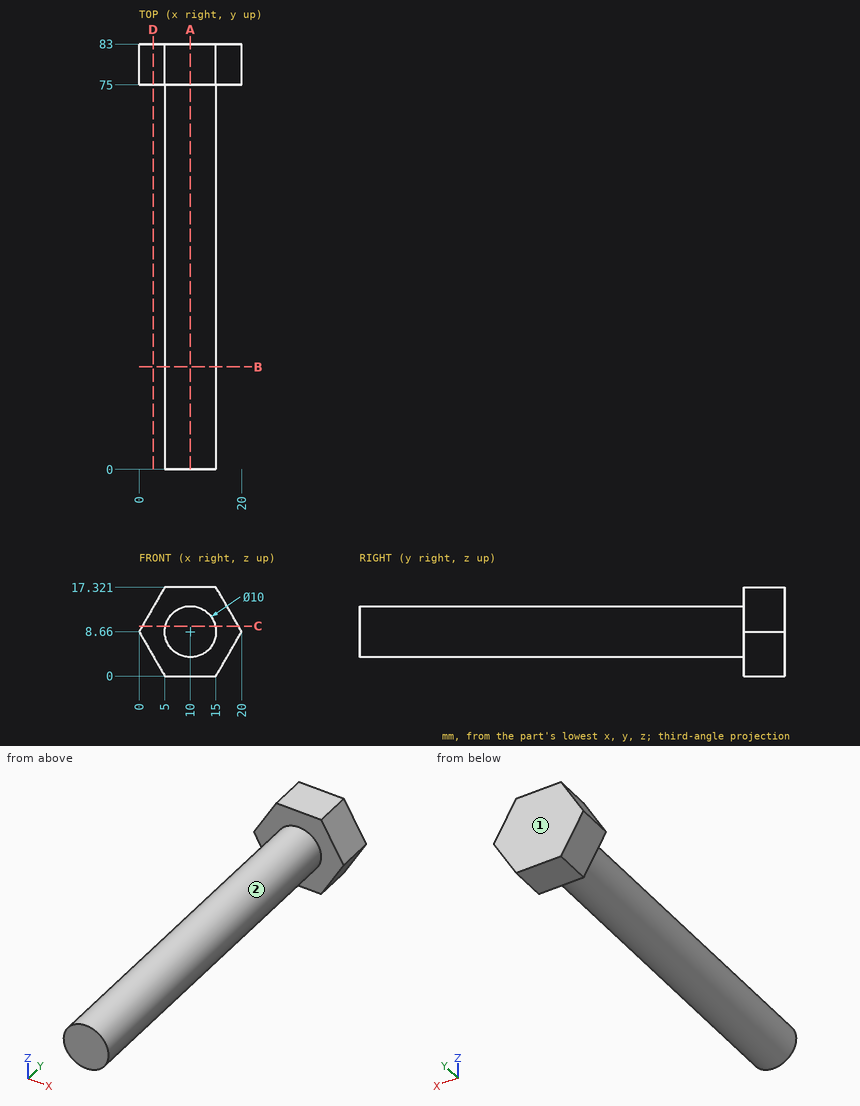
The drawing under review shows one solid part. Ordinate dimensions are in mm from its lowest x, y, z. A direction names the side the tool comes from. Round coordinates to 2 decimals unless told otherwise and drop trailing zeros. Loops run counter-clockwise (first coordinate to the right, second up) from the corner with the lowest first, then second, coordinate; pieces in that order, holes last.
Item 1: Take a section at C-C (z = 9.75). Write out the cut boundary in (x, y), then the cut area to 3 significant figures.
Determined:
outline: (0.63, 75) - (5.12, 75) - (5.12, 0) - (14.88, 0) - (14.88, 75) - (19.37, 75) - (19.37, 83) - (0.63, 83) - close
area: 882 mm2
Item 2: Take a section at A-A (x = 10). Write out the cut boundary in (y, z).
Determined:
outline: (0, 3.66) - (75, 3.66) - (75, 0) - (83, 0) - (83, 17.32) - (75, 17.32) - (75, 13.66) - (0, 13.66) - close
Item 3: Take a section at B-B (y = 20). Write out the cut boundary in (x, z).
Determined:
outline: circle Ø10 at (10, 8.66)
Item 4: Clearance check with flat-ended pins moving along their axes: pin 1 Ø10 at (x, y) = (16.5, 9.5) entering from -Z; pin 2 Ø8 at (y, z) = (27, 7) entering from -X; pin 3 Ø6 at (y, z) = (12.5, 4.5) entering from -X. State where each tip first meets the part, or that it passes through.
Determined:
pin 1: stops at z = 3.89
pin 2: stops at x = 5
pin 3: stops at x = 5.14
Item 5: For line 1 (Y direction, x = 4, z = 9.25); line 2 (X direction, y = 62.5, z = 6.5); line 3 (Z direction, x = 7.25, y = 7.5) (1 decimal), list the stretches that pass through material, from the lowest coordinate up.
Determined:
line 1: y = 75 to 83
line 2: x = 5.49 to 14.51
line 3: z = 4.5 to 12.8
Item 6: For the marked faces 1 and 2, list the 3-axis set-ups (+Z, -Z, +X, -X, +Y, -Y) from which the entire face can be reached by the end or side of a thin tool; tool diameter is ignored.
Determined:
face 1: +Z, -Z, +X, -X, +Y
face 2: -Y
Item 7: Take a section at D-D (x = 2.75). Write out the cut boundary in (y, z), then the cut area to 3 significant figures.
Determined:
outline: (75, 3.9) - (83, 3.9) - (83, 13.42) - (75, 13.42) - close
area: 76.2 mm2
